Check sheet for the modelled part. Datum: model origin and axes. Units: mm. A direction names the side the tool comes from. Round coordinates to 2 decimals unless told otherwise and drop trailing zeros. Order: outer loops, then holes, each group sorted by start corner. A loop starts at its lowest first (then second) coordinate and runs counter-clockwise, first axis right, second up. Notation, with made-up numbers: (28, 49) -> (67, 49) arc R24 ccw to (67, 60) -> close; hole circle Ø6 at (67, 37). An arc over 180 degrees is marked (long way). Answer in a Markdown table with one row per item. Add a question column.
1. Material ranges on L1, parallel to Z at x = 0, y = 4.5; L2, parallel to Z at x = 0, y = 2.25; L3, parallel to Z at x = -1.75, y = -4.5, recorded low to high. Write a range as from..to.
2. Depth check by flat-ended pin: P1, Ø5, axis at x = -4.5, z = 7, coming from the -Y side; P2, Ø6, axis at y = 4.5, z = 5, coming from the +X side; P3, Ø2, axis at x = 0.5, z = 4, coming from the +Y side; P4, Ø2, axis at y = -3, z = 2.5, coming from the +X side. Enter the tip coordinate at first touch or a pass-through.
3. Sectioned sample at A-A, the plane x = 0. Record the boundary of the cut face in (y, z).
4. Sectioned sample at C-C, the plane y = 4.25. Record the boundary of the cut face in (x, z).
5. Sectioned sample at B-B, the plane y = -2. Record the boundary of the cut face in (x, z).
6. Access from +Z, -Z, +X, -X, +Y, -Y to the whole of each face (thin tool, end or side, straight path). Record for faces 1 (the flat face through (3, -1, 6.5)), 2 (the cylindrical face through (3.07, 5.9, 3.2)), 3 (the cylindrical face through (0.748, 3.279, 2.274)).
7. Draft check along Z on faces 4 (the flat face through (0, 0, 3)), 5 (the cylindrical face through (-3, 0, 8)), 6 (the flat face through (0, 0, 0)), 7 (the flat face through (0, 0, 10.549)). Enter one of: +Z half, -Z half, draft (parallel to the pull), parting line (faces both ways), or undercut.
8. Sectioned sample at D-D, the plane z = 5. Record the boundary of the cut face in (x, y), then the cut area to 3 significant figures.
Autodesk Inventor part; units mm, degrees
ref_plane "Work Plane1" through (-6.65, 6.65, 6.5) normal (0, 1, 0) x (1, 0, 0)
ref_plane "YZ Plane" through (0, 0, 0) normal (1, 0, 0) x (0, 1, 0)
ref_plane "XZ Plane" through (0, 0, 0) normal (0, 1, 0) x (-1, 0, 0)
sketch "Sketch1" plane through (0, 0, 0) normal (0, 0, 1) x (1, 0, 0)
  circle A0 centre (0, 0) radius 6.65
  dimension "d0" = 13.3
extrude "Extrusion1" add sketch "Sketch1" along normal blind 6.5
ref_plane "Work Plane1" through (-6.65, 6.65, 6.5) normal (0, 1, 0) x (1, 0, 0)
sketch "Sketch3" plane through (-6.65, 6.65, 6.5) normal (0, 1, 0) x (1, 0, 0)
  circle A0 centre (6.65, 3.25) radius 1.2
  dimension "d9" = 2.4
hole "Hole1" at (0, 6.65, 3.25) direction (0, -1, 0) diameter 2.459 depth 6.65
sketch "Sketch4" plane through (0, 0, 6.5) normal (0, 0, 1) x (1, 0, 0)
  circle A0 centre (0, 0) radius 6.65
  circle A1 centre (0, 0) radius 3
  dimension "d17" = 6
extrude "Extrusion3" add sketch "Sketch4" along normal blind 4.049 contours A1
properties part number "hridel kuzelova kolecka"
Answer key:
| question | item | result |
|---|---|---|
| 1 | L1 | z = 0..2.02, 4.48..6.5 |
| 1 | L2 | z = 0..2.02, 4.48..10.55 |
| 1 | L3 | z = 0..6.5 |
| 2 | P1 | stops at y = -6.33 |
| 2 | P2 | stops at x = 6.48 |
| 2 | P3 | stops at y = 6.65 |
| 2 | P4 | stops at x = 6.34 |
| 3 | outline | (-6.65, 0) -> (6.65, 0) -> (6.65, 2.02) -> (0, 2.02) -> (0, 4.48) -> (6.65, 4.48) -> (6.65, 6.5) -> (3, 6.5) -> (3, 10.55) -> (-3, 10.55) -> (-3, 6.5) -> (-6.65, 6.5) -> close |
| 4 | outline | (-5.11, 0) -> (5.11, 0) -> (5.11, 6.5) -> (-5.11, 6.5) -> close; hole circle Ø2.46 at (0, 3.25) |
| 5 | outline | (-6.34, 0) -> (6.34, 0) -> (6.34, 6.5) -> (2.24, 6.5) -> (2.24, 10.55) -> (-2.24, 10.55) -> (-2.24, 6.5) -> (-6.34, 6.5) -> close |
| 6 | face 1 | +Z |
| 6 | face 2 | +Z, -Z |
| 6 | face 3 | +Y |
| 7 | face 4 | undercut |
| 7 | face 5 | draft |
| 7 | face 6 | -Z half |
| 7 | face 7 | +Z half |
| 8 | outline | circle Ø13.3 at (0, 0) |
| 8 | area | 139 mm² |
